```python
from build123d import *

# Parameters (mm, degrees)
F0_R     = 40.5
F1_DEPTH = 7.5
F3_SIZE  = 20
F2_R     = 2.5
F4_DEPTH = 25
F5_R     = 2.5
F6_DEPTH = 10
F7_R     = 2.5
F8_DEPTH = 10


# Not quite as in the source:
# - a feature names something its author has since deleted; it is built from what else it names


with BuildPart() as f1:
    # F0 (on Top) → F1 (new body)
    with BuildSketch(Plane.XY):
        with BuildLine():
            Line((43, 47), (43, 55))
            Line((43, 55), (-43, 55))
            Line((-43, 55), (-43, 47))
            ThreePointArc((-43, 47), (-40.1715728753, 45.8284271247), (-39, 43))
            ThreePointArc((-39, 43), (-43, 39), (-47, 43))
            Line((-47, 43), (-85, 43))
            Line((-85, 43), (-85, -43))
            Line((-85, -43), (-47, -43))
            ThreePointArc((-47, -43), (-43, -39), (-39, -43))
            ThreePointArc((-39, -43), (-40.1715728753, -45.8284271247), (-43, -47))
            Line((-43, -47), (-43, -55))
            Line((-43, -55), (41, -55))
            Line((41, -55), (85, -55))
            Line((85, -55), (85, 43))
            Line((85, 43), (47, 43))
            ThreePointArc((47, 43), (40.1715728753, 40.1715728753), (43, 47))
        make_face()
        with BuildLine():
            ThreePointArc((52, -41), (48.7781745931, -48.7781745931), (41, -52))
            ThreePointArc((41, -52), (33.2218254069, -33.2218254069), (52, -41))
        make_face(mode=Mode.SUBTRACT)
        Circle(F0_R, mode=Mode.SUBTRACT)
        with BuildLine():
            Line((85, 43), (85, 55))
            Line((85, 55), (43, 55))
            Line((43, 55), (43, 47))
            ThreePointArc((43, 47), (45.8284271247, 45.8284271247), (47, 43))
            Line((47, 43), (85, 43))
        make_face()
        with BuildLine():
            Line((-85, -55), (-43, -55))
            Line((-43, -55), (-43, -47))
            ThreePointArc((-43, -47), (-45.8284271247, -45.8284271247), (-47, -43))
            Line((-47, -43), (-85, -43))
            Line((-85, -43), (-85, -55))
        make_face()
        with BuildLine():
            Line((-43, 47), (-43, 55))
            Line((-43, 55), (-85, 55))
            Line((-85, 55), (-85, 43))
            Line((-85, 43), (-47, 43))
            ThreePointArc((-47, 43), (-45.8284271247, 45.8284271247), (-43, 47))
        make_face()
    extrude(amount=F1_DEPTH)

    # F3
    f3_edges = [f1.edges().sort_by_distance(p)[0] for p in [
        (85, -55, 3.75),
        (-85, -55, 3.75),
        (-85, 55, 3.75),
        (85, 55, 3.75),
    ]]
    chamfer(f3_edges, length=F3_SIZE)

    # F2 (on face) → F4 (cut)
    with BuildSketch(Plane(origin=(0, 0, 0), x_dir=(1, 0, 0), z_dir=(0, 0, -1))):
        with Locations((77, -25)):
            Circle(F2_R)
        with Locations((77, 25)):
            Circle(F2_R)
        with Locations((-77, 25)):
            Circle(F2_R)
        with Locations((-77, -25)):
            Circle(F2_R)
    extrude(amount=-F4_DEPTH, mode=Mode.SUBTRACT)

    # F5 (on face) → F6 (cut)
    with BuildSketch(Plane.XZ.offset(55)):
        with Locations((-43, 3.75)):
            Circle(F5_R)
        with Locations((41, 3.75)):
            Circle(F5_R)
    extrude(amount=-F6_DEPTH, mode=Mode.SUBTRACT)

    # F7 (on face) → F8 (cut)
    with BuildSketch(Plane(origin=(0, 55, 0), x_dir=(-1, 0, 0), z_dir=(0, 1, 0))):
        with Locations((-43, 3.75)):
            Circle(F7_R)
        with Locations((43, 3.75)):
            Circle(F7_R)
    extrude(amount=-F8_DEPTH, mode=Mode.SUBTRACT)


solid = f1.part
```
For this review, take the finished solid that the model builds, in its own axes (mm). A direction names the side the tool comes from. Coordinates: 2 decimals unless noted, no trailing zeros. Loops run counter-clockwise (first coordinate to the right, second up) from the corner with the lowest first, then second, coordinate; pieces in that order, holes last.
1. Mouldability with a two-part tool opening along Y and no side actions: class faces 4 (the cylindrical face through (-40.502, 50.623, 3.86)), 5 (the cylindrical face through (75.16, -26.69, 3.7)), 6 (the flat face through (-75, 45, 4)) as +Y half, -Y half, draft (parallel to the pull), parting line (faces both ways), or undercut.
2. Add section D-D, the plane z = 3.75. Count the separate pieces of the cut face and the enclosed holes in it, then the cut area to 3 significant figures.
3. Add section B-B, the plane x = 0. Give the boundary of the cut face in (y, z), then the cut area to 4 significant figures.
4. Insertion check: P1, Ø4.5, axis at x = -77, y = 25, coming from the +Z side; P2, Ø3, axis at x = 41, z = 3.75, coming from the -Y side; P3, Ø4.5, axis at x = -43, z = 3.75, coming from the -Y side; P4, Ø4, axis at x = 67, y = 23.5, coming from the -Z side. Each pin has a flat end and moves straight along its axis. Give the tip position at first contact, or say it passes through.
5. For faces 1 (the flat face through (-75, -45, 4)), 2 (the cylindrical face through (45.498, 50.623, 3.86)), 3 (the cylindrical face through (-45.498, -50.623, 3.86)), list the 3-axis set-ups (+Z, -Z, +X, -X, +Y, -Y) from which the entire face can be reached by the end or side of a thin tool; tool diameter is ignored.
6. Add section C-C, the plane y = 30. Give the boundary of the cut face in (x, z), then the cut area to 3 significant figures.
7. For line 1 (Y direction, x = -77, z = 3); line 2 (X direction, y = -49, z = 3); line 3 (X direction, y = -49.75, z = 3.75), list the stretches that pass through material, from the lowest coordinate up.
8. Add section A-A, the plane x = 77. Give the boundary of the cut face in (y, z), then the cut area to 3 significant figures.
Result:
1. face 4: draft
1. face 5: undercut
1. face 6: +Y half
2. separate pieces: 1
2. enclosed holes: 5
2. area: 12,000 mm2
3. outline: (-55, 0) - (-40.5, 0) - (-40.5, 7.5) - (-55, 7.5) - close; (40.5, 0) - (55, 0) - (55, 7.5) - (40.5, 7.5) - close
3. area: 217.5 mm2
4. P1: passes through
4. P2: stops at y = -30.1
4. P3: stops at y = -39.69
4. P4: stops at z = 0
5. face 1: +Z, -Z, -X, -Y
5. face 2: +Y
5. face 3: -Y
6. outline: (-85, 0) - (-27.21, 0) - (-27.21, 7.5) - (-85, 7.5) - close; (27.21, 0) - (85, 0) - (85, 7.5) - (27.21, 7.5) - close
6. area: 867 mm2
7. line 1: y = -43 to -27.5, -22.5 to 22.5, 27.5 to 43
7. line 2: x = -71 to -45.38, -40.62 to 33.45, 48.55 to 71
7. line 3: x = -70.25 to -45.5, -40.5 to 34.33, 47.67 to 70.25
8. outline: (-43, 0) - (-27.5, 0) - (-27.5, 7.5) - (-43, 7.5) - close; (-22.5, 0) - (22.5, 0) - (22.5, 7.5) - (-22.5, 7.5) - close; (27.5, 0) - (43, 0) - (43, 7.5) - (27.5, 7.5) - close
8. area: 570 mm2
